For this review, take the finished solid that the model builds, in its own axes (mm). A direction names the side the tool comes from. Give positions to 0.01 mm unless a question says otherwise; leave off trailing zeros. Write each loop counter-clockwise with the first axis right and the second up, starting at its lowest first coordinate (ties: lowest second). Pieces come first, ordered by that corner, then holes.
Autodesk Inventor part; units mm, degrees
ref_plane "YZ Plane" through (0, 0, 0) normal (1, 0, 0) x (0, 1, 0)
ref_plane "XZ Plane" through (0, 0, 0) normal (0, 1, 0) x (-1, 0, 0)
ref_plane "XY Plane" through (0, 0, 0) normal (0, 0, 1) x (1, 0, 0)
sketch "Sketch1" plane through (0, 0, 0) normal (0, 0, 1) x (1, 0, 0)
  circle A0 centre (0, 0) radius 3.9624
  dimension "d0" = 7.9248
extrude "Extrusion1" add sketch "Sketch1" along normal blind 4.826
sketch "Sketch2" plane through (0, 0, 0) normal (0, 0, -1) x (-1, 0, 0)
  circle A0 centre (0, 0) radius 3.9624
  circle A1 centre (0, 0) radius 2.413
  dimension "d3" = 4.826
extrude "Extrusion2" add sketch "Sketch2" along normal blind 15.875 contours A1
sketch "Sketch3" plane through (0, 0, 4.826) normal (0, 0, 1) x (1, 0, 0)
  circle A0 centre (0, 0) radius 3.9624
  line L0 (-1.1457, 1.9844) -> (1.1457, 1.9844)
  line L1 (1.1457, 1.9844) -> (2.2914, 0)
  line L2 (2.2914, 0) -> (1.1457, -1.9844)
  line L3 (1.1457, -1.9844) -> (-1.1457, -1.9844)
  line L4 (-1.1457, -1.9844) -> (-2.2914, 0)
  line L5 (-2.2914, 0) -> (-1.1457, 1.9844)
  dimension "d6" = 3.9688
extrude "Extrusion3" cut sketch "Sketch3" against normal blind 3.175 contours L0 L1 L2 L3 L4 L5
thread "Thread1"
chamfer "Chamfer1" distance 0.508 angle 45 1 edges at (2.413, 0, -15.875)
chamfer "Chamfer2" distance 0.508 angle 45 1 edges at (-3.9624, 0, 4.826)
properties part number "10-32 x1000" material "Steel"
(1) We need section A-A (x = 0). Write out the cut boundary in (y, z) (3 decimals).
(2) Tool access review of faces 5 (the cylindrical face through (1.915, 1.468, -7.576)), 6 (the flat face through (1.727, -0.978, 3.261)), 7 (the flat face through (0, 0, -15.875)): name each direction out of +Z, -Z, +X, -X, +Y, -Y from which nothing blocks a thin tool from reaching the whole face with its end or side.
(3) We need section C-C (z = 0.5). Write out the cut boundary in (x, y), and give its area (3 significant figures).
(4) For L1, parallel to Z at x = -2.25, y = 1.5; L2, parallel to Y at x = 0.75, z = -3.75; L3, parallel to Z at x = -0.75, y = -0.5 (3 decimals), list the stretches that pass through material, from the lowest coordinate up.
(5) Clearance check with flat-ended pins moving along their axes: pin 1 Ø2 at (x, y) = (1, 0) entering from +Z; pin 2 Ø1 at (x, z) = (0, -9.5) entering from -Y; pin 3 Ø1.5 at (x, z) = (1.5, -3) entering from -Y. State where each tip first meets the part, or that it passes through.
(6) The part is to be moulded in two halves that separate along X. For faces 1 (the flat face through (2, 2, 0)), 2 (the flat face through (-1.727, 0.978, 3.261)), 3 (the flat face through (0, 0, 1.651)), 4 (the cylindrical face through (-0.52, -3.93, 2.13)), say which applies: +X half, -X half, draft (parallel to the pull), parting line (faces both ways), or undercut.
(7) We need section B-B (z = -6.75). Write out the cut boundary in (x, y), and give its area (3 significant figures).
The answers:
1. outline: (-3.962, 0) - (-2.413, 0) - (-2.413, -15.367) - (-1.905, -15.875) - (1.905, -15.875) - (2.413, -15.367) - (2.413, 0) - (3.962, 0) - (3.962, 4.318) - (3.454, 4.826) - (1.984, 4.826) - (1.984, 1.651) - (-1.984, 1.651) - (-1.984, 4.826) - (-3.454, 4.826) - (-3.962, 4.318) - close
2. face 5: -Z
2. face 6: +Z
2. face 7: -Z, +X, -X, +Y, -Y
3. outline: circle Ø7.92 at (0, 0)
3. area: 49.3 mm2
4. L1: z = 0 to 4.83
4. L2: y = -2.29 to 2.29
4. L3: z = -15.875 to 1.651
5. pin 1: stops at z = 1.65
5. pin 2: stops at y = -2.41
5. pin 3: stops at y = -2.29
6. face 1: draft
6. face 2: undercut
6. face 3: undercut
6. face 4: parting line
7. outline: circle Ø4.83 at (0, 0)
7. area: 18.3 mm2
